The model under review builds one solid part; all positions refer to its coordinate system, in mm. Face numbers are marked on the shaded views. Coordinates: 2 decimals unless noted, no trailing zeros. Write each loop counter-clockwise with the first axis right and the second up, starting at its lowest first coordinate (ties: lowest second). Pieces come first, ordered by that corner, then holes.
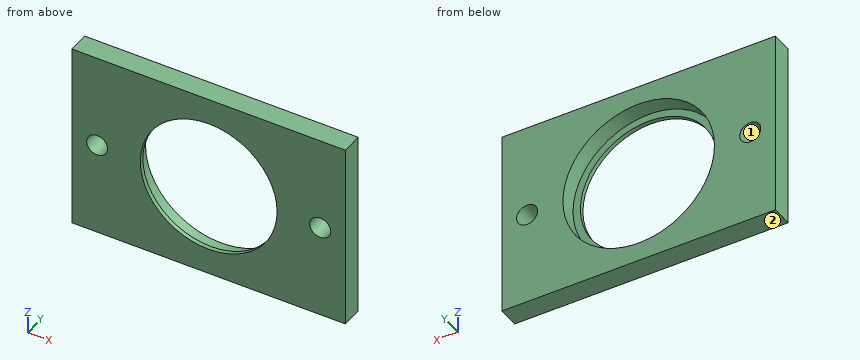
Solid Edge part; units mm, degrees
sketch "Sketch1" plane through (0, 0, 0) normal (0, -1, 0) x (1, 0, 0)
  line L0 (65, -45) -> (65, 45)
  line L1 (65, 45) -> (-65, 45)
  line L2 (-65, 45) -> (-65, -45)
  line L3 (-65, -45) -> (65, -45)
extrude "Protrusion1" add sketch "Sketch1" along normal blind 10
sketch "Sketch2" plane through (0, 0, 0) normal (0, 1, 0) x (1, 0, 0)
  circle A0 centre (0, 0) radius 36
extrude "ExtrudedCutout_1" cut sketch "Sketch2" against normal blind 8
sketch "Sketch3" plane through (0, 0, 0) normal (0, 1, 0) x (1, 0, 0)
  circle A0 centre (-53, 0) radius 5
  circle A1 centre (53, 0) radius 5
extrude "Cutout1" cut sketch "Sketch3" against normal up to next
sketch "Sketch4" plane through (0, -8, 0) normal (0, 1, 0) x (1, 0, 0)
  circle A0 centre (0, 0) radius 32.5
extrude "Cutout2" cut sketch "Sketch4" against normal up to next
Item 1: Take a section at B-B, the plane z = 0. Write out the cut boundary in (x, y).
Solved:
outline: (-65, -10) - (-58, -10) - (-58, 0) - (-65, 0) - close; (-48, -10) - (-32.5, -10) - (-32.5, -8) - (-36, -8) - (-36, 0) - (-48, 0) - close; (32.5, -10) - (48, -10) - (48, 0) - (36, 0) - (36, -8) - (32.5, -8) - close; (58, -10) - (65, -10) - (65, 0) - (58, 0) - close
Item 2: Take a section at C-C, the plane y = -2.5. Write out the cut boundary in (x, z), plus the area to 3 significant figures.
Solved:
outline: (-65, -45) - (65, -45) - (65, 45) - (-65, 45) - close; hole circle Ø10 at (-53, 0); hole circle Ø72 at (0, 0); hole circle Ø10 at (53, 0)
area: 7,470 mm2
Item 3: To check wall thickness, follow line 1 along X through (y, z) = (-9.1, 0); line 2 along X through (y, z) = (-7.5, 0.5); line 3 along Z through (x, y) = (53, -3.5). State the ranges of each line that lie inside material, in increasing order.
Solved:
line 1: x = -65 to -58, -48 to -32.5, 32.5 to 48, 58 to 65
line 2: x = -65 to -57.97, -48.03 to -36, 36 to 48.03, 57.97 to 65
line 3: z = -45 to -5, 5 to 45
Item 4: Take a section at A-A, the plane x = 0. Write out the cut boundary in (y, z).
Solved:
outline: (-10, -45) - (0, -45) - (0, -36) - (-8, -36) - (-8, -32.5) - (-10, -32.5) - close; (-10, 32.5) - (-8, 32.5) - (-8, 36) - (0, 36) - (0, 45) - (-10, 45) - close
Item 5: Mouldability with a two-part tool opening along X and no side actions: class the marked faces 1 and 2 as pulls with the +X half, pulls with the -X half, needs draft (parallel to the pull), parting line crosses it, or undercut.
Solved:
face 1: undercut
face 2: needs draft
Item 6: Take a section at D-D, the plane z = 18. Write out the cut boundary in (x, y), plus the area to 3 significant figures.
Solved:
outline: (-65, -10) - (-27.06, -10) - (-27.06, -8) - (-31.18, -8) - (-31.18, 0) - (-65, 0) - close; (27.06, -10) - (65, -10) - (65, 0) - (31.18, 0) - (31.18, -8) - (27.06, -8) - close
area: 693 mm2
